CAD build for the part. Positions are in the model's coordinates, mm. Coordinates: 2 decimals unless noted, no trailing zeros. Order: outer loops, then holes, each group sorted by start corner. A loop starts at its lowest first (then second) coordinate and runs counter-clockwise, first axis right, second up. Notation, with made-up numbers: (-15, 2.5) - (-2, 2.5) arc R25 cw to (-2, 31.5) - close; hole circle Ø2 at (61, 11). An arc over 180 degrees is marked (long way). Return JSON: item names as keys, results as strings.
from build123d import *

# Parameters (mm, degrees)
F0_R        = 5
F0_R_2      = 4
F3_C1_SIZE2 = 0.6516126864
F3_C1_SIZE  = 0.5
F3_C2_SIZE2 = 0.5
F3_C2_SIZE  = 0.6516126864


with BuildPart() as f2:
    # F2: sweep along a path in F1
    with BuildLine(Plane.XZ) as f2_path:
        Line((0, 0), (0, 21))
        ThreePointArc((0, 21), (-5.2720779386, 33.7279220614), (-18, 39))
        Line((-18, 39), (-39, 39))
    # F0 (on Top) → F2 (sweep)
    with BuildSketch(Plane.XY):
        Circle(F0_R)
        Circle(F0_R_2, mode=Mode.SUBTRACT)
    sweep(path=f2_path.line)

    # F3: chamfer of 0.5 x 0.6516126864 on 2 edges, made by hand

    # F3_c1
    f3_c1_edges = [f2.edges().sort_by_distance(p)[0] for p in [
        (-5, 0, 0),
    ]]
    f3_c1_side = f2.faces().sort_by_distance((-5, 0, 0.01))[0]
    chamfer(f3_c1_edges, length=F3_C1_SIZE, length2=F3_C1_SIZE2, reference=f3_c1_side)

    # F3_c2
    f3_c2_edges = [f2.edges().sort_by_distance(p)[0] for p in [
        (-39, 0, 34),
    ]]
    f3_c2_side = f2.faces().sort_by_distance((-38.99, 0, 34))[0]
    chamfer(f3_c2_edges, length=F3_C2_SIZE, length2=F3_C2_SIZE2, reference=f3_c2_side)


solid = f2.part
Item 1: Band-saw the part on A-A, the plane y = 0. List the corners of the cut face in (x, z).
Findings below:
{"outline": "(-39, 34.5) - (-38.35, 34) - (-18, 34) arc R13 cw to (-5, 21) - (-5, 0.5) - (-4.35, 0) - (-4, 0) - (-4, 21) arc R14 ccw to (-18, 35) - (-39, 35) - close; (-39, 43) - (-18, 43) arc R22 cw to (4, 21) - (4, 0) - (4.35, 0) - (5, 0.5) - (5, 21) arc R23 ccw to (-18, 44) - (-38.35, 44) - (-39, 43.5) - close"}
Item 2: Drop flat-ended pins along their axis: P1, Ø1, axis at x = -2.5, z = 15, coming from the +Y side; P2, Ø3, axis at x = -21.5, y = -0.5, coming from the -Z side; P3, Ø1.5, axis at x = -16.5, z = 36, coming from the +Y side. Give the stop position or say it passes through.
Findings below:
{"P1": "stops at y = 4.58", "P2": "stops at z = 34", "P3": "stops at y = 4.5"}
Item 3: Wall check: L1, parallel to Z at x = -32, y = 0; L2, parallel to Y at x = -30, z = 39; L3, parallel to Z at x = -10.5, y = -1.75. Give the ranges that are in metal, low to high. Write a range as [from, to].
Findings below:
{"L1": "z = [34, 35], [43, 44]", "L2": "y = [-5, -4], [4, 5]", "L3": "z = [32, 33.3], [41.25, 42.41]"}
Item 4: Band-saw the part on B-B, the plane x = -36. List the corners of the cut face in (y, z).
Findings below:
{"outline": "circle Ø10 at (0, 39); hole circle Ø8 at (0, 39)"}
Item 5: Mould opens along Y. For faces 1 (the cylindrical face through (-0.867, -3.905, 10.647)), 2 (the flat face through (-39, 3, 42)), 3 (the cylindrical face through (-28, 0, 34)), 4 (the cylindrical face through (-28.6, -2.4, 35.8)) say: released by +Y, released by -Y, zero draft, split by the parting line, or undercut.
Findings below:
{"face 1": "undercut", "face 2": "zero draft", "face 3": "split by the parting line", "face 4": "undercut"}
Item 6: Band-saw the part on C-C, the plane z = 13.5. List the corners of the cut face in (x, y), then the cut area to 3 significant figures.
Findings below:
{"outline": "circle Ø10 at (0, 0); hole circle Ø8 at (0, 0)", "area": "28.3 mm²"}
